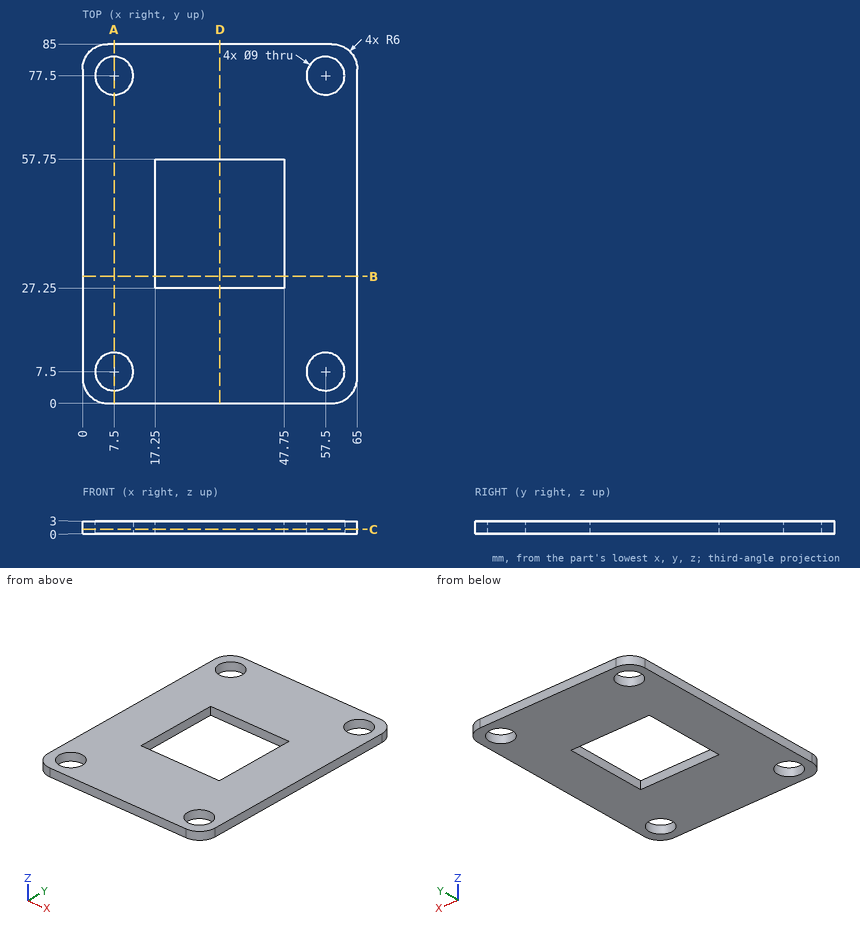
Print and shaded views of the part. All mm, measured from the part's lowest x, y and z. Round coordinates to 2 decimals unless told otherwise and drop trailing zeros. Order: outer loops, then holes, each group sorted by start corner. A loop starts at its lowest first (then second) coordinate and runs counter-clockwise, first axis right, second up.
Q1. Slice it at A-A (x = 7.5). Write the cut outline in (y, z), and give its area (3 significant figures).
Q2. Slice it at D-D (x = 32.5). Write the cut outline in (y, z), and give its area (4 significant figures).
Q3. Slice it at C-C (z = 1.1). Write the cut outline in (x, y), and give its area (3 significant figures).
Q4. Wall check: L1, parallel to Y at x = 57.5, z = 2.2; L2, parallel to Y at x = 28, z = 1.5; L3, parallel to Y at x = 4, z = 1.75. Give the ranges that are in metal, low to high.
Q5. Slice it at B-B (y = 30). Write the cut outline in (x, z).
Results below:
1. outline: (0, 0) - (3, 0) - (3, 3) - (0, 3) - close; (12, 0) - (73, 0) - (73, 3) - (12, 3) - close; (82, 0) - (85, 0) - (85, 3) - (82, 3) - close
1. area: 201 mm2
2. outline: (0, 0) - (27.25, 0) - (27.25, 3) - (0, 3) - close; (57.75, 0) - (85, 0) - (85, 3) - (57.75, 3) - close
2. area: 163.5 mm2
3. outline: (0, 6) arc R6 ccw to (6, 0) - (59, 0) arc R6 ccw to (65, 6) - (65, 79) arc R6 ccw to (59, 85) - (6, 85) arc R6 ccw to (0, 79) - close; hole circle Ø9 at (7.5, 7.5); hole circle Ø9 at (7.5, 77.5); hole (17.25, 27.25) - (47.75, 27.25) - (47.75, 57.75) - (17.25, 57.75) - close; hole circle Ø9 at (57.5, 7.5); hole circle Ø9 at (57.5, 77.5)
3. area: 4,310 mm2
4. L1: y = 0 to 3, 12 to 73, 82 to 85
4. L2: y = 0 to 27.25, 57.75 to 85
4. L3: y = 0.34 to 4.67, 10.33 to 74.67, 80.33 to 84.66
5. outline: (0, 0) - (17.25, 0) - (17.25, 3) - (0, 3) - close; (47.75, 0) - (65, 0) - (65, 3) - (47.75, 3) - close
